from build123d import *

# Parameters (mm, degrees)
SKETCH1_W           = 82.9
SKETCH1_H           = 82.9
BOSS_EXTRUDE1_DEPTH = 0.5
SKETCH2_R           = 3.6
CUT_EXTRUDE1_DEPTH  = 59.62128453
FILLET1_R           = 2
SKETCH3_R           = 1.6
CUT_EXTRUDE2_DEPTH  = 10
SKETCH4_R           = 2
CUT_EXTRUDE3_DEPTH  = 10
SKETCH7_W           = 8.2
SKETCH7_H           = 28
CUT_EXTRUDE5_DEPTH  = 10
FILLET3_R           = 0.5


with BuildPart() as part:
    # Sketch1 → Boss-Extrude1 (new body)
    with BuildSketch(Plane(origin=(0, 0, 0), x_dir=(1, 0, 0), z_dir=(0, 1, 0))):
        Rectangle(SKETCH1_W, SKETCH1_H)
    extrude(amount=BOSS_EXTRUDE1_DEPTH)

    # Sketch2 → Cut-Extrude1 (cut, through all)
    with BuildSketch(Plane(origin=(0, 0.5, 0), x_dir=(1, 0, 0), z_dir=(0, 1, 0))):
        with Locations(Location((-30, 30, 0), (0, 0, 270))):
            Circle(SKETCH2_R)
        with Locations(Location((30, 30, 0), (0, 0, 270))):
            Circle(SKETCH2_R)
        with Locations(Location((30, -30, 0), (0, 0, 270))):
            Circle(SKETCH2_R)
        with Locations(Location((-30, -30, 0), (0, 0, 270))):
            Circle(SKETCH2_R)
    extrude(amount=-CUT_EXTRUDE1_DEPTH, mode=Mode.SUBTRACT)

    # Fillet1
    fillet1_edges = [part.edges().sort_by_distance(p)[0] for p in [
        (41.45, 0.25, 41.45),
        (-41.45, 0.25, 41.45),
        (-41.45, 0.25, -41.45),
        (41.45, 0.25, -41.45),
    ]]
    fillet(fillet1_edges, radius=FILLET1_R)

    # Sketch3 → Cut-Extrude2 (cut)
    with BuildSketch(Plane(origin=(0, 0.5, 0), x_dir=(1, 0, 0), z_dir=(0, 1, 0))):
        with Locations(Location((-36.5, 36.5, 0), (0, 0, 270))):
            Circle(SKETCH3_R)
        with Locations(Location((36.5, 36.5, 0), (0, 0, 270))):
            Circle(SKETCH3_R)
        with Locations(Location((36.5, -36.5, 0), (0, 0, 270))):
            Circle(SKETCH3_R)
        with Locations(Location((-36.5, -36.5, 0), (0, 0, 270))):
            Circle(SKETCH3_R)
    extrude(amount=-CUT_EXTRUDE2_DEPTH, mode=Mode.SUBTRACT)

    # Sketch4 → Cut-Extrude3 (cut)
    with BuildSketch(Plane(origin=(0, 0.5, 0), x_dir=(1, 0, 0), z_dir=(0, 1, 0))):
        with Locations(Location((19.999999567, 31.499795659, 0), (0, 0, 270))):
            Circle(SKETCH4_R)
        with Locations(Location((19.999999567, 22.999799474, 0), (0, 0, 270))):
            Circle(SKETCH4_R)
    extrude(amount=-CUT_EXTRUDE3_DEPTH, mode=Mode.SUBTRACT)

    # Sketch7 → Cut-Extrude5 (cut)
    with BuildSketch(Plane(origin=(0, 0.5, 0), x_dir=(1, 0, 0), z_dir=(0, 1, 0))):
        with Locations((9.09999852, 20.7799998)):
            Rectangle(SKETCH7_W, SKETCH7_H)
    extrude(amount=-CUT_EXTRUDE5_DEPTH, mode=Mode.SUBTRACT)

    # Fillet3
    fillet3_edges = [part.edges().sort_by_distance(p)[0] for p in [
        (13.19999852, 0.25, -34.7799998),
        (13.19999852, 0.25, -6.7799998),
        (4.99999852, 0.25, -6.7799998),
        (4.99999852, 0.25, -34.7799998),
    ]]
    fillet(fillet3_edges, radius=FILLET3_R)


solid = part.part
Design review of the part built by this model. Coordinates are the model's own, in mm. Give positions to 0.01 mm unless a question says otherwise; leave off trailing zeros. Loops run counter-clockwise (first coordinate to the right, second up) from the corner with the lowest first, then second, coordinate; pieces in that order, holes last. Notation, with made-up numbers: M 27,-26.75 L 35,-26.75 A22 cw 35,-15.75 Z; hole C 25,68 d2. An arc over 180 degrees is marked long. Write item = value, one per line.
Q1. Insertion check: pin 1 (5 mm diameter, centred on x = 33, z = -28.5, fed in from -Y). The pin has a flat end and moves straight along its axis. Give the tip position at first contact, or say it passes through.
Output values:
pin_1 = 0
Q2. We need section C-C (y = 0.3). Count the separate pieces of the cut face and the enclosed holes in it, plus the area to 3 significant figures.
Output values:
separate_pieces = 1
enclosed_holes = 11
area = 6,420 mm^2
Q3. We need section B-B (z = 30). Give the boundary of the cut face in (x, y), plus the area to 4 significant figures.
Output values:
outline = M -41.45,0 L -33.6,0 L -33.6,0.5 L -41.45,0.5 Z; M -26.4,0 L 26.4,0 L 26.4,0.5 L -26.4,0.5 Z; M 33.6,0 L 41.45,0 L 41.45,0.5 L 33.6,0.5 Z
area = 34.25 mm^2
Q4. To check wall thickness, follow line 1 (X direction, y = 0.45, z = 36.5); line 2 (Z direction, x = 20, y = 0.2); line 3 (Z direction, x = -35.5, y = 0.35). State the ranges of each line that lie inside material, in increasing order. Write a range as [from, to].
Output values:
line_1 = [-41.45, -38.1], [-34.9, 34.9], [38.1, 41.45]
line_2 = [-41.45, -33.5], [-29.5, -25], [-21, 41.45]
line_3 = [-41.45, -37.75], [-35.25, 35.25], [37.75, 41.45]
Q5. Draft analysis for pull direction X (two halves, no side actions). For faces 1 (the cylindrical face through (-40.88, 0.25, -40.85)), 2 (the cylindrical face through (35.08, 0.25, -35.76)), 3 (the cylindrical face through (40.85, 0.25, 40.88)), state which applies: +X half, -X half, draft (parallel to the pull), parting line (faces both ways), or undercut.
Output values:
face_1 = -X half
face_2 = undercut
face_3 = +X half
Q6. We need section A-A (x = 36.5). Give the boundary of the cut face in (y, z), plus the area to 4 significant figures.
Output values:
outline = M 0,-41.45 L 0.5,-41.45 L 0.5,-38.1 L 0,-38.1 Z; M 0,-34.9 L 0.5,-34.9 L 0.5,34.9 L 0,34.9 Z; M 0,38.1 L 0.5,38.1 L 0.5,41.45 L 0,41.45 Z
area = 38.25 mm^2
